from build123d import *

# Parameters (mm, degrees)
SKETCH_1_W             = 72
SKETCH_1_H             = 150
EXTRUDE_1_DEPTH        = 1
SKETCH_2_R             = 1.4
CUT_EXTRUDE_1_DEPTH    = 2
PATTERN_LINEAR_1_COUNT = 2
PATTERN_LINEAR_1_PITCH = 5
PATTERN_LINEAR_2_COUNT = 2
PATTERN_LINEAR_2_PITCH = 5
SKETCH_9_W             = 72
SKETCH_9_H             = 7.5
CUT_EXTRUDE_4_DEPTH    = 5.5
EXTRUDE_5_DEPTH        = 2
SKETCH_12_W            = 72
SKETCH_12_H            = 48.96667592
CUT_EXTRUDE_5_DEPTH    = 10
SKETCH_14_R            = 1.65
CUT_EXTRUDE_6_DEPTH    = 10
SKETCH_15_W            = 3.2
SKETCH_15_H            = 10.2
CUT_EXTRUDE_7_DEPTH    = 10
SKETCH_16_R            = 1.3
CUT_EXTRUDE_8_DEPTH    = 10
SKETCH_17_R            = 1.65
CUT_EXTRUDE_9_DEPTH    = 10
FILLET_1_R             = 2
SKETCH_18_W            = 20.5
SKETCH_18_H            = 43
CUT_EXTRUDE_10_DEPTH   = 10
CUT_EXTRUDE_11_DEPTH   = 10
FILLET_2_R             = 1.3
SKETCH_20_W            = 45
SKETCH_20_H            = 26.033324079
CUT_EXTRUDE_12_DEPTH   = 10
FILLET_3_R             = 2
SKETCH_21_W            = 5
SKETCH_21_H            = 20.5
CUT_EXTRUDE_13_DEPTH   = 10
FILLET_4_R             = 2
SKETCH_22_W            = 156
SKETCH_22_H            = 2.5
CUT_EXTRUDE_14_DEPTH   = 3
FILLET_5_R             = 3


with BuildPart() as part:
    # 草图1 → 凸台-拉伸1 (new body, symmetric)
    with BuildSketch(Plane.XY):
        Rectangle(SKETCH_1_W, SKETCH_1_H)
    extrude(amount=EXTRUDE_1_DEPTH, both=True)

    # 草图2 → 切除-拉伸1 (cut)
    with BuildSketch(Plane(origin=(0, 0, -1), x_dir=(-1, 0, 0), z_dir=(0, 0, -1))):
        with Locations((-27, -12.3)):
            Circle(SKETCH_2_R)
        with Locations((27, -12.3)):
            Circle(SKETCH_2_R)
        with Locations((27, 59.7)):
            Circle(SKETCH_2_R)
        with Locations((-27, 59.7)):
            Circle(SKETCH_2_R)
    cut_extrude_1 = extrude(amount=-CUT_EXTRUDE_1_DEPTH, mode=Mode.SUBTRACT)

    # 阵列(线性)1: 切除-拉伸1 ×2
    with Locations(*[(0, -i * PATTERN_LINEAR_1_PITCH, 0) for i in range(1, PATTERN_LINEAR_1_COUNT)]):
        add(cut_extrude_1, mode=Mode.SUBTRACT)

    # 阵列(线性)2: 切除-拉伸1 ×2
    with Locations(*[(0, i * PATTERN_LINEAR_2_PITCH, 0) for i in range(1, PATTERN_LINEAR_2_COUNT)]):
        add(cut_extrude_1, mode=Mode.SUBTRACT)

    # 草图9 → 切除-拉伸4 (cut)
    with BuildSketch(Plane.XY.offset(1)):
        with Locations((0, -71.25)):
            Rectangle(SKETCH_9_W, SKETCH_9_H)
    extrude(amount=-CUT_EXTRUDE_4_DEPTH, mode=Mode.SUBTRACT)

    # 草图11 → 凸台-拉伸5 (add)
    with BuildSketch(Plane(origin=(0, 0, -1), x_dir=(-1, 0, 0), z_dir=(0, 0, -1))):
        Polygon((-36, 36), (-78, -43.01666204), (-36, -43.01666204), align=None)
        Polygon((36, -43.01666204), (36, 36), (78, -43.01666204), align=None)
    extrude(amount=-EXTRUDE_5_DEPTH)

    # 草图12 → 切除-拉伸5 (cut)
    with BuildSketch(Plane.XY.offset(1)):
        with Locations((0, -67.5)):
            Rectangle(SKETCH_12_W, SKETCH_12_H)
    extrude(amount=-CUT_EXTRUDE_5_DEPTH, mode=Mode.SUBTRACT)

    # 草图14 → 切除-拉伸6 (cut)
    with BuildSketch(Plane(origin=(0, 0, -1), x_dir=(-1, 0, 0), z_dir=(0, 0, -1))):
        with Locations((-49.82296811, -0.658849754)):
            Circle(SKETCH_14_R)
        with Locations((-59.209976564, -18.319089624)):
            Circle(SKETCH_14_R)
        with Locations((49.82296811, -0.658849754)):
            Circle(SKETCH_14_R)
        with Locations((59.209976564, -18.319089624)):
            Circle(SKETCH_14_R)
    extrude(amount=-CUT_EXTRUDE_6_DEPTH, mode=Mode.SUBTRACT)

    # 草图15 → 切除-拉伸7 (cut)
    with BuildSketch(Plane(origin=(0, 0, -1), x_dir=(-1, 0, 0), z_dir=(0, 0, -1))):
        with Locations((30.75, 37)):
            Rectangle(SKETCH_15_W, SKETCH_15_H)
        with Locations((-30.7673157, 37)):
            Rectangle(SKETCH_15_W, SKETCH_15_H)
    extrude(amount=-CUT_EXTRUDE_7_DEPTH, mode=Mode.SUBTRACT)

    # 草图16 → 切除-拉伸8 (cut)
    with BuildSketch(Plane(origin=(0, 0, -1), x_dir=(-1, 0, 0), z_dir=(0, 0, -1))):
        with Locations((-29.1673157, 40.8)):
            Circle(SKETCH_16_R)
        with Locations((-32.3673157, 40.8)):
            Circle(SKETCH_16_R)
        with Locations((-32.3673157, 33.2)):
            Circle(SKETCH_16_R)
        with Locations((-29.1673157, 33.2)):
            Circle(SKETCH_16_R)
        with Locations((29.1673157, 33.2)):
            Circle(SKETCH_16_R)
        with Locations((32.3673157, 33.2)):
            Circle(SKETCH_16_R)
        with Locations((32.3673157, 40.8)):
            Circle(SKETCH_16_R)
        with Locations((29.1673157, 40.8)):
            Circle(SKETCH_16_R)
    extrude(amount=-CUT_EXTRUDE_8_DEPTH, mode=Mode.SUBTRACT)

    # 草图17 → 切除-拉伸9 (cut)
    with BuildSketch(Plane(origin=(0, 0, -1), x_dir=(-1, 0, 0), z_dir=(0, 0, -1))):
        with Locations((-30.7673157, 47.6)):
            Circle(SKETCH_17_R)
        with Locations((30.7673157, 47.6)):
            Circle(SKETCH_17_R)
    extrude(amount=-CUT_EXTRUDE_9_DEPTH, mode=Mode.SUBTRACT)

    # 圆角1
    fillet_1_edges = [part.edges().sort_by_distance(p)[0] for p in [
        (-36, 75, 0),
        (36, 75, 0),
    ]]
    fillet(fillet_1_edges, radius=FILLET_1_R)

    # 草图18 → 切除-拉伸10 (cut)
    with BuildSketch(Plane(origin=(0, 0, -1), x_dir=(-1, 0, 0), z_dir=(0, 0, -1))):
        with Locations((12.25, 48.5)):
            Rectangle(SKETCH_18_W, SKETCH_18_H)
        with Locations((-12.25, 48.5)):
            Rectangle(SKETCH_18_W, SKETCH_18_H)
        with Locations((-12.25, 1.5)):
            Rectangle(SKETCH_18_W, SKETCH_18_H)
        with Locations((12.25, 1.5)):
            Rectangle(SKETCH_18_W, SKETCH_18_H)
    extrude(amount=-CUT_EXTRUDE_10_DEPTH, mode=Mode.SUBTRACT)

    # 草图19 → 切除-拉伸11 (cut)
    with BuildSketch(Plane(origin=(0, 0, -1), x_dir=(-1, 0, 0), z_dir=(0, 0, -1))):
        Polygon((-31.5, -7.895665687), (-48.573384423, -7.895665687), (-64.052168457, -37.01666204), (-31.5, -37.01666204), align=None)
        Polygon((-31.5, 24.225330666), (-46.978784034, -4.895665687), (-31.5, -4.895665687), align=None)
        Polygon((31.5, 24.225330666), (31.5, -4.895665687), (46.978784034, -4.895665687), align=None)
        Polygon((48.573384423, -7.895665687), (31.5, -7.895665687), (31.5, -37.01666204), (64.052168457, -37.01666204), align=None)
    extrude(amount=-CUT_EXTRUDE_11_DEPTH, mode=Mode.SUBTRACT)

    # 圆角2
    fillet_2_edges = [part.edges().sort_by_distance(p)[0] for p in [
        (-2, 23, 0),
        (-22.5, 23, 0),
        (-22.5, -20, 0),
        (-2, -20, 0),
        (2, 23, 0),
        (2, -20, 0),
        (22.5, -20, 0),
        (22.5, 23, 0),
        (2, 70, 0),
        (2, 27, 0),
        (22.5, 27, 0),
        (22.5, 70, 0),
        (-2, 70, 0),
        (-22.5, 70, 0),
        (-22.5, 27, 0),
        (-2, 27, 0),
        (-48.573384423, -7.895665687, 0),
        (-64.052168457, -37.01666204, 0),
        (-31.5, -37.01666204, 0),
        (-31.5, -7.895665687, 0),
        (-31.5, 24.225330666, 0),
        (-46.978784034, -4.895665687, 0),
        (-31.5, -4.895665687, 0),
        (31.5, -4.895665687, 0),
        (46.978784034, -4.895665687, 0),
        (31.5, 24.225330666, 0),
        (31.5, -7.895665687, 0),
        (31.5, -37.01666204, 0),
        (64.052168457, -37.01666204, 0),
        (48.573384423, -7.895665687, 0),
    ]]
    fillet(fillet_2_edges, radius=FILLET_2_R)

    # 草图20 → 切除-拉伸12 (cut)
    with BuildSketch(Plane(origin=(0, 0, -1), x_dir=(-1, 0, 0), z_dir=(0, 0, -1))):
        with Locations((0, -43.01666204)):
            Rectangle(SKETCH_20_W, SKETCH_20_H)
    extrude(amount=-CUT_EXTRUDE_12_DEPTH, mode=Mode.SUBTRACT)

    # 圆角3
    fillet_3_edges = [part.edges().sort_by_distance(p)[0] for p in [
        (22.5, -30, 0),
        (-22.5, -30, 0),
    ]]
    fillet(fillet_3_edges, radius=FILLET_3_R)

    # 草图21 → 切除-拉伸13 (cut)
    with BuildSketch(Plane(origin=(0, 0, -1), x_dir=(-1, 0, 0), z_dir=(0, 0, -1))):
        with Locations((-33.5, 64.75)):
            Rectangle(SKETCH_21_W, SKETCH_21_H)
        with Locations((33.5, 64.75)):
            Rectangle(SKETCH_21_W, SKETCH_21_H)
    extrude(amount=-CUT_EXTRUDE_13_DEPTH, mode=Mode.SUBTRACT)

    # 圆角4
    fillet_4_edges = [part.edges().sort_by_distance(p)[0] for p in [
        (31, 54.5, 0),
        (31, 75, 0),
        (36, 54.5, 0),
        (-36, 54.5, 0),
        (-31, 54.5, 0),
        (-31, 75, 0),
    ]]
    fillet(fillet_4_edges, radius=FILLET_4_R)

    # 草图22 → 切除-拉伸14 (cut, through all)
    with BuildSketch(Plane(origin=(0, 0, -1), x_dir=(-1, 0, 0), z_dir=(0, 0, -1))):
        with Locations((0, -41.76666204)):
            Rectangle(SKETCH_22_W, SKETCH_22_H)
    extrude(amount=-CUT_EXTRUDE_14_DEPTH, mode=Mode.SUBTRACT)

    # 圆角5
    fillet_5_edges = [part.edges().sort_by_distance(p)[0] for p in [
        (22.5, -40.51666204, 0),
        (76.671166343, -40.51666204, 0),
        (-76.671166343, -40.51666204, 0),
        (-22.5, -40.51666204, 0),
    ]]
    fillet(fillet_5_edges, radius=FILLET_5_R)


solid = part.part
For this review, take the finished solid that the model builds, in its own axes (mm). A direction names the side the tool comes from. Round coordinates to 2 decimals unless told otherwise and drop trailing zeros. Write each loop counter-clockwise with the first axis right and the second up, starting at its lowest first coordinate (ties: lowest second). Pieces come first, ordered by that corner, then holes. Notation, with made-up numbers: (-29.75, 28.5) - (23.25, 28.5) arc R19 ccw to (23.25, 44.5) - close; hole circle Ø11 at (72.5, -6.5). An arc over 180 degrees is marked (long way). Write item = value, one per line. Start each with the question number.
1. Draft analysis for pull direction Y (two halves, no side actions). For faces 4 (the face through (54.896, 0.45, -0.014)), 5 (the face through (-74.228, -39.099, -0.014)), 6 (the face through (23.4, -39.66, 0.01)), 7 (the face through (-40.04, 8.16, -0.01)), state which applies: released by +Y, released by -Y, zero draft, split by the parting line, or undercut.
2. Consider section B-B on y = 47.6. State the section outline as (x, z) points, plus the area to 3 significant figures.
3. Consider section C-C on x = 53. State the section outline as (y, z) points.
4. Wall thickness on L1, parallel to X at y = 51, z = 0.75; L2, parallel to X at y = 39, z = 0.35; L3, parallel to Y at x = 29, z = -0.45: over which ranges is each line inside the solid? List them lowest first.
5. Consider section A-A on x = 16.5. State the section outline as (y, z) points.
6. For pin 1 Ø1 at (y, z) = (58, -0.5) entering from +X; pin 2 Ø2 at (x, y) = (30.77, 47.6) entering from +Z; pin 3 Ø1.1 at (x, z) = (33.5, 0.5) entering from +Y; pin 4 Ø4.5 at (x, y) = (27, -7.3) entering from -Z, all flat-tipped, find the tip position at first contact; note any pin that passes through.
7. For faces 1 (the face through (55.89, -21.66, -0.01)), 2 (the face through (-23.355, -39.615, 0.014)), 3 (the face through (0, 5, -1)), list the 3-axis set-ups (+Z, -Z, +X, -X, +Y, -Y) from which the entire face can be reached by the end or side of a thin tool; tool diameter is ignored.
8. Consider section D-D on z = 0.1. Give the number of separate pieces and of enclosed holes in the cut face, plus the area to 3 significant figures.
Evaluation:
q1.face_4 = released by +Y
q1.face_5 = split by the parting line
q1.face_6 = released by -Y
q1.face_7 = undercut
q2.outline = (-36, -1) - (-32.42, -1) - (-32.42, 1) - (-36, 1) - close; (-29.12, -1) - (-22.5, -1) - (-22.5, 1) - (-29.12, 1) - close; (-2, -1) - (2, -1) - (2, 1) - (-2, 1) - close; (22.5, -1) - (29.12, -1) - (29.12, 1) - (22.5, 1) - close; (32.42, -1) - (36, -1) - (36, 1) - (32.42, 1) - close
q2.area = 48.8 mm2
q3.outline = (-40.52, -1) - (-37.02, -1) - (-37.02, 1) - (-40.52, 1) - close; (-16.22, -1) - (4.02, -1) - (4.02, 1) - (-16.22, 1) - close
q4.L1 = -36 to -22.5, -2 to 2, 22.5 to 36
q4.L2 = -36 to -32.35, -29.15 to -22.5, -2 to 2, 22.5 to 29.17, 32.37 to 36
q4.L3 = -40.52 to 31.91, 34.49 to 39.51, 42.09 to 75
q5.outline = (-30, -1) - (-20, -1) - (-20, 1) - (-30, 1) - close; (23, -1) - (27, -1) - (27, 1) - (23, 1) - close; (70, -1) - (75, -1) - (75, 1) - (70, 1) - close
q6.pin_1 = 31
q6.pin_2 = through
q6.pin_3 = 54.5
q6.pin_4 = -1
q7.face_1 = +Z, -Z
q7.face_2 = +Z, -Z, -Y
q7.face_3 = -Z, +X, -X, +Y, -Y
q8.separate_pieces = 1
q8.enclosed_holes = 28
q8.area = 5,120 mm2
